Verification items for the finished model (mm, model axes). A direction names the side the tool comes from. Give positions to 0.01 mm unless a question says otherwise; leave off trailing zeros. Order: outer loops, then holes, each group sorted by start corner. A loop starts at its lowest first (then second) coordinate and runs counter-clockwise, first axis right, second up.
from build123d import *

# Parameters (mm, degrees)
SKETCH1_R           = 1.5
BOSS_EXTRUDE1_DEPTH = 2.5
BOSS_EXTRUDE5_DEPTH = 8


with BuildPart() as part:
    # Sketch1 → Boss-Extrude1 (new body)
    # profile 1 of 5: a face of its own
    with BuildSketch(Plane(origin=(0, 0, 0), x_dir=(1, 0, 0), z_dir=(0, 1, 0))):
        with BuildLine():
            ThreePointArc((5.938658614, 8.045640675), (2.651650429, 2.651650429), (8.045640675, 5.938658614))
            ThreePointArc((8.045640675, 5.938658614), (7.071067812, 7.071067812), (5.938658614, 8.045640675))
        make_face()
        with Locations(Location((4.949747468, 4.949747468, 0), (0, 0, 270))):
            Circle(SKETCH1_R, mode=Mode.SUBTRACT)
    # profile 2 of 5: a face of its own
    with BuildSketch(Plane(origin=(0, 0, 0), x_dir=(1, 0, 0), z_dir=(0, 1, 0))):
        with BuildLine():
            ThreePointArc((8.045640675, -5.938658614), (10, 0), (8.045640675, 5.938658614))
            ThreePointArc((8.045640675, 5.938658614), (2.651650429, 2.651650429), (5.938658614, 8.045640675))
            ThreePointArc((5.938658614, 8.045640675), (0, 10), (-5.938658614, 8.045640675))
            ThreePointArc((-5.938658614, 8.045640675), (-2.651650429, 2.651650429), (-8.045640675, 5.938658614))
            ThreePointArc((-8.045640675, 5.938658614), (-10, 0), (-8.045640675, -5.938658614))
            ThreePointArc((-8.045640675, -5.938658614), (-2.651650429, -2.651650429), (-5.938658614, -8.045640675))
            ThreePointArc((-5.938658614, -8.045640675), (0, -10), (5.938658614, -8.045640675))
            ThreePointArc((5.938658614, -8.045640675), (2.651650429, -2.651650429), (8.045640675, -5.938658614))
        make_face()
        with BuildLine():
            Line((-4.722131518, -1), (-4.722131518, 1))
            Line((-4.722131518, 1), (-2.722131518, 1))
            ThreePointArc((-2.722131518, 1), (2.9, 0), (-2.722131518, -1))
            Line((-2.722131518, -1), (-4.722131518, -1))
        make_face(mode=Mode.SUBTRACT)
    # profile 3 of 5: a face of its own
    with BuildSketch(Plane(origin=(0, 0, 0), x_dir=(1, 0, 0), z_dir=(0, 1, 0))):
        with BuildLine():
            ThreePointArc((5.938658614, -8.045640675), (7.071067812, -7.071067812), (8.045640675, -5.938658614))
            ThreePointArc((8.045640675, -5.938658614), (2.651650429, -2.651650429), (5.938658614, -8.045640675))
        make_face()
        with Locations(Location((4.949747468, -4.949747468, 0), (0, 0, 270))):
            Circle(SKETCH1_R, mode=Mode.SUBTRACT)
    # profile 4 of 5: a face of its own
    with BuildSketch(Plane(origin=(0, 0, 0), x_dir=(1, 0, 0), z_dir=(0, 1, 0))):
        with BuildLine():
            ThreePointArc((-8.045640675, 5.938658614), (-2.651650429, 2.651650429), (-5.938658614, 8.045640675))
            ThreePointArc((-5.938658614, 8.045640675), (-7.071067812, 7.071067812), (-8.045640675, 5.938658614))
        make_face()
        with Locations(Location((-4.949747468, 4.949747468, 0), (0, 0, 270))):
            Circle(SKETCH1_R, mode=Mode.SUBTRACT)
    # profile 5 of 5: a face of its own
    with BuildSketch(Plane(origin=(0, 0, 0), x_dir=(1, 0, 0), z_dir=(0, 1, 0))):
        with BuildLine():
            ThreePointArc((-8.045640675, -5.938658614), (-7.071067812, -7.071067812), (-5.938658614, -8.045640675))
            ThreePointArc((-5.938658614, -8.045640675), (-2.651650429, -2.651650429), (-8.045640675, -5.938658614))
        make_face()
        with Locations(Location((-4.949747468, -4.949747468, 0), (0, 0, 270))):
            Circle(SKETCH1_R, mode=Mode.SUBTRACT)
    extrude(amount=BOSS_EXTRUDE1_DEPTH)

    # Sketch1_14 → Boss-Extrude5 (add)
    with BuildSketch(Plane(origin=(0, 0, 0), x_dir=(1, 0, 0), z_dir=(0, 1, 0))):
        with BuildLine():
            ThreePointArc((8.045640675, -5.938658614), (10, 0), (8.045640675, 5.938658614))
            ThreePointArc((8.045640675, 5.938658614), (2.651650429, 2.651650429), (5.938658614, 8.045640675))
            ThreePointArc((5.938658614, 8.045640675), (0, 10), (-5.938658614, 8.045640675))
            ThreePointArc((-5.938658614, 8.045640675), (-2.651650429, 2.651650429), (-8.045640675, 5.938658614))
            ThreePointArc((-8.045640675, 5.938658614), (-10, 0), (-8.045640675, -5.938658614))
            ThreePointArc((-8.045640675, -5.938658614), (-2.651650429, -2.651650429), (-5.938658614, -8.045640675))
            ThreePointArc((-5.938658614, -8.045640675), (0, -10), (5.938658614, -8.045640675))
            ThreePointArc((5.938658614, -8.045640675), (2.651650429, -2.651650429), (8.045640675, -5.938658614))
        make_face()
        with BuildLine():
            Line((-4.722131518, -1), (-4.722131518, 1))
            Line((-4.722131518, 1), (-2.722131518, 1))
            ThreePointArc((-2.722131518, 1), (2.9, 0), (-2.722131518, -1))
            Line((-2.722131518, -1), (-4.722131518, -1))
        make_face(mode=Mode.SUBTRACT)
    extrude(amount=BOSS_EXTRUDE5_DEPTH)


solid = part.part
(1) Section check A-A, the plane y = 3.25. Enter the section's corners in (x, z).
Solved:
outline: (-8.05, -5.94) arc R3.25 cw (long way) to (-5.94, -8.05) arc R10 ccw to (5.94, -8.05) arc R3.25 cw (long way) to (8.05, -5.94) arc R10 ccw to (8.05, 5.94) arc R3.25 cw (long way) to (5.94, 8.05) arc R10 ccw to (-5.94, 8.05) arc R3.25 cw (long way) to (-8.05, 5.94) arc R10 ccw to start; hole (-4.72, -1) - (-2.72, -1) arc R2.9 ccw (long way) to (-2.72, 1) - (-4.72, 1) - close
(2) Section check C-C, the plane x = 0. Enter the section's corners in (y, z).
Solved:
outline: (0, -10) - (8, -10) - (8, -2.9) - (0, -2.9) - close; (0, 2.9) - (8, 2.9) - (8, 10) - (0, 10) - close
(3) Scan lines: line 1 (Z direction, x = -4, y = 4.75); line 2 (Z direction, x = 6, y = 2.25); line 3 (X direction, y = 1.5, z = -5.25). Record each from-to range of solid material in increasing order.
Solved:
line 1: z = -9.17 to -8.06, -1.84 to -1, 1 to 1.84, 8.06 to 9.17
line 2: z = -8 to -6.02, -3.88 to 3.88, 6.02 to 8
line 3: x = -8.51 to -6.42, -3.48 to 3.48, 6.42 to 8.51
(4) Section check B-B, the plane z = 0. Enter the section's corners in (x, y).
Solved:
outline: (-10, 0) - (-4.72, 0) - (-4.72, 8) - (-10, 8) - close; (2.9, 0) - (10, 0) - (10, 8) - (2.9, 8) - close
(5) Release check for a two-part mould opening along Z. For faces 4 (the flat face through (2.1, 8, -2.4)), 5 (the cylindrical face through (-3.463, 1.232, -5.145)) record: pulls with the +Z half, pulls with the -Z half, needs draft (parallel to the pull), parting line crosses it, or undercut.
Solved:
face 4: needs draft
face 5: undercut
(6) Section check D-D, the plane y = 1. Enter the section's corners in (x, z), then the cut area to 3 significant figures.
Solved:
outline: circle Ø20 at (0, 0); hole circle Ø3 at (-4.95, -4.95); hole circle Ø3 at (-4.95, 4.95); hole (-4.72, -1) - (-2.72, -1) arc R2.9 ccw (long way) to (-2.72, 1) - (-4.72, 1) - close; hole circle Ø3 at (4.95, -4.95); hole circle Ø3 at (4.95, 4.95)
area: 256 mm2
(7) Set-up check for faces 1 (the cylindrical face through (2.568, 5.212, 2.739)), 2 (the flat face through (-4, 4, -1)), 3 (the flat face through (2.1, 0, -2.4)): record each of +Z, -Z, +X, -X, +Y, -Y from which the full face is reachable in a straight line by a thin tool's end or side.
Solved:
face 1: +Y
face 2: +Y, -Y
face 3: +Z, -Z, +X, -X, -Y
(8) Go/stop test with flat-tipped pins: pin 1 (2 mm diameter, centred on x = 6.5, z = 5.5, fed in from +Y); pin 2 (5 mm diameter, centred on x = 0, z = 0, fed in from +Y); pin 3 (3 mm diameter, centred on y = 3, z = 6.5, fed in from -X); pin 4 (1.6 mm diameter, centred on x = -4, y = 5.5, fed in from +Z). Record where each tip stops, or that it passes through.
Solved:
pin 1: stops at y = 2.5
pin 2: passes through
pin 3: stops at x = -8.66
pin 4: stops at z = 9.47
